Can you work these out from the model? Positions are in its coordinate system, mm. A direction names the side the tool comes from. Round coordinates to 2 decimals unless told otherwise and drop trailing zeros. Loops run counter-clockwise (first coordinate to the right, second up) from the corner with the lowest first, then second, coordinate; pieces in that order, holes last.
```python
from build123d import *

# Parameters (mm, degrees)
SKETCH4_W                      = 106
SKETCH4_H                      = 24
BOSS_EXTRUDE2_DEPTH            = 13
CUT_EXTRUDE3_START             = -9.7
SKETCH25_W                     = 106
SKETCH25_H                     = 8.1
CUT_EXTRUDE3_DEPTH             = 110.207903902
M5_CLEARANCE_HOLE1_D           = 5.5
SKETCH39_R                     = 4.2
CUT_EXTRUDE5_DEPTH             = 3.2
MIRROR3_START                  = -40.65
MIRROR3_OUTLINE_W              = 106
MIRROR3_OUTLINE_H              = 13
MIRROR3_OUTLINE_R              = 2.75
MIRROR3_DEPTH                  = 7.948683024
MIRROR3_START_2                = -24.601316976
MIRROR3_2_OUTLINE_W            = 106
MIRROR3_2_OUTLINE_H            = 13
MIRROR3_2_OUTLINE_R            = 4.2
MIRROR3_2_DEPTH                = 7.951316976
MIRROR3_START_3                = -32.701316976
MIRROR3_3_OUTLINE_W            = 106
MIRROR3_3_OUTLINE_H            = 3.3
MIRROR3_3_DEPTH                = 12.851316976
MIRROR3_4_OUTLINE_R            = 2.75
MIRROR3_4_DEPTH                = 4.751316976
M4_CLEARANCE_HOLE2_D           = 4.5
SKETCH31_W                     = 88
SKETCH31_H                     = 7
CUT_EXTRUDE4_DEPTH             = 7
SKETCH32_W                     = 6.6
SKETCH32_H                     = 7.948683024
BOSS_EXTRUDE3_DEPTH            = 10
SKETCH37_W                     = 6.6
SKETCH37_H                     = 7.948683024
BOSS_EXTRUDE4_DEPTH            = 10
M4_CLEARANCE_HOLE1_D           = 4.5
M4_CLEARANCE_HOLE1_ON_FACE_2_D = 4.5
SKETCH42_R                     = 4.75
CUT_EXTRUDE9_DEPTH             = 7
SKETCH43_R                     = 4.75
CUT_EXTRUDE10_DEPTH            = 7


# Read off the part's stored shape, not the designer's step: Mirror3
with BuildPart() as part:
    # Sketch4 → Boss-Extrude2 (new body)
    with BuildSketch(Plane.XY):
        with Locations((-36.891047602, -28.65)):
            Rectangle(SKETCH4_W, SKETCH4_H)
    extrude(amount=-BOSS_EXTRUDE2_DEPTH)

    # Sketch25 → Cut-Extrude3 (cut)
    with BuildSketch(Plane.XY.offset(CUT_EXTRUDE3_START)):
        with Locations((-36.891047602, -28.651316976)):
            Rectangle(SKETCH25_W, SKETCH25_H)
    extrude(amount=CUT_EXTRUDE3_DEPTH, mode=Mode.SUBTRACT)

    # M5 Clearance Hole1 (through all)
    with Locations(Plane(origin=(-74.391047602, -16.65, -5.55), x_dir=(0, 0, 1), z_dir=(0, 1, 0))):
        with Locations((0, 0), (0, 25), (0, 75), (0, 50)):
            Hole(M5_CLEARANCE_HOLE1_D / 2)

    # Sketch39 → Cut-Extrude5 (cut)
    with BuildSketch(Plane(origin=(0, -16.65, 0), x_dir=(1, 0, 0), z_dir=(0, 1, 0))):
        with Locations(Location((0.608952398, 5.55, 0), (0, 0, 270))):
            Circle(SKETCH39_R)
        with Locations(Location((-24.391047602, 5.55, 0), (0, 0, 270))):
            Circle(SKETCH39_R)
        with Locations(Location((-49.391047602, 5.55, 0), (0, 0, 270))):
            Circle(SKETCH39_R)
        with Locations(Location((-74.391047602, 5.55, 0), (0, 0, 270))):
            Circle(SKETCH39_R)
    extrude(amount=-CUT_EXTRUDE5_DEPTH, mode=Mode.SUBTRACT)

    # Mirror3 outline → Mirror3 (add)
    with BuildSketch(Plane(origin=(0, 0, 0), x_dir=(1, 0, 0), z_dir=(0, 1, 0)).offset(MIRROR3_START)):
        with Locations((-36.891047602, 19.5)):
            Rectangle(MIRROR3_OUTLINE_W, MIRROR3_OUTLINE_H)
        with Locations((0.608952398, 20.45)):
            Circle(MIRROR3_OUTLINE_R, mode=Mode.SUBTRACT)
        with Locations((-24.391047602, 20.45)):
            Circle(MIRROR3_OUTLINE_R, mode=Mode.SUBTRACT)
        with Locations((-49.391047602, 20.45)):
            Circle(MIRROR3_OUTLINE_R, mode=Mode.SUBTRACT)
        with Locations((-74.391047602, 20.45)):
            Circle(MIRROR3_OUTLINE_R, mode=Mode.SUBTRACT)
    extrude(amount=MIRROR3_DEPTH)

    # Mirror3 2 outline → Mirror3 2 (add)
    with BuildSketch(Plane(origin=(0, 0, 0), x_dir=(1, 0, 0), z_dir=(0, 1, 0)).offset(MIRROR3_START_2)):
        with Locations((-36.891047602, 19.5)):
            Rectangle(MIRROR3_2_OUTLINE_W, MIRROR3_2_OUTLINE_H)
        with Locations((0.608952398, 20.45)):
            Circle(MIRROR3_2_OUTLINE_R, mode=Mode.SUBTRACT)
        with Locations((-24.391047602, 20.45)):
            Circle(MIRROR3_2_OUTLINE_R, mode=Mode.SUBTRACT)
        with Locations((-49.391047602, 20.45)):
            Circle(MIRROR3_2_OUTLINE_R, mode=Mode.SUBTRACT)
        with Locations((-74.391047602, 20.45)):
            Circle(MIRROR3_2_OUTLINE_R, mode=Mode.SUBTRACT)
    extrude(amount=MIRROR3_2_DEPTH)

    # Mirror3 3 outline → Mirror3 3 (add)
    with BuildSketch(Plane(origin=(0, 0, 0), x_dir=(1, 0, 0), z_dir=(0, 1, 0)).offset(MIRROR3_START_3)):
        with Locations((-36.891047602, 14.65)):
            Rectangle(MIRROR3_3_OUTLINE_W, MIRROR3_3_OUTLINE_H)
    extrude(amount=MIRROR3_3_DEPTH)

    # Mirror3 4 outline → Mirror3 4 (add)
    # profile 1 of 4: a face of its own
    with BuildSketch(Plane(origin=(0, 0, 0), x_dir=(1, 0, 0), z_dir=(0, 1, 0)).offset(MIRROR3_START_2)):
        with BuildLine():
            Line((-0.037190001, 16.3), (1.255094797, 16.3))
            ThreePointArc((1.255094797, 16.3), (0.608952398, 24.65), (-0.037190001, 16.3))
        make_face()
        with Locations((0.608952398, 20.45)):
            Circle(MIRROR3_4_OUTLINE_R, mode=Mode.SUBTRACT)
    # profile 2 of 4: a face of its own
    with BuildSketch(Plane(origin=(0, 0, 0), x_dir=(1, 0, 0), z_dir=(0, 1, 0)).offset(MIRROR3_START_2)):
        with BuildLine():
            ThreePointArc((-73.744905203, 16.3), (-74.391047602, 24.65), (-75.037190001, 16.3))
            Line((-75.037190001, 16.3), (-73.744905203, 16.3))
        make_face()
        with Locations((-74.391047602, 20.45)):
            Circle(MIRROR3_4_OUTLINE_R, mode=Mode.SUBTRACT)
    # profile 3 of 4: a face of its own
    with BuildSketch(Plane(origin=(0, 0, 0), x_dir=(1, 0, 0), z_dir=(0, 1, 0)).offset(MIRROR3_START_2)):
        with BuildLine():
            Line((-25.037190001, 16.3), (-23.744905203, 16.3))
            ThreePointArc((-23.744905203, 16.3), (-24.391047602, 24.65), (-25.037190001, 16.3))
        make_face()
        with Locations((-24.391047602, 20.45)):
            Circle(MIRROR3_4_OUTLINE_R, mode=Mode.SUBTRACT)
    # profile 4 of 4: a face of its own
    with BuildSketch(Plane(origin=(0, 0, 0), x_dir=(1, 0, 0), z_dir=(0, 1, 0)).offset(MIRROR3_START_2)):
        with BuildLine():
            ThreePointArc((-48.744905203, 16.3), (-49.391047602, 24.65), (-50.037190001, 16.3))
            Line((-50.037190001, 16.3), (-48.744905203, 16.3))
        make_face()
        with Locations((-49.391047602, 20.45)):
            Circle(MIRROR3_4_OUTLINE_R, mode=Mode.SUBTRACT)
    extrude(amount=MIRROR3_4_DEPTH)

    # M4 Clearance Hole2 (through all)
    with Locations(Plane(origin=(11.108952398, -40.65, -13), x_dir=(0, 0, -1), z_dir=(0, -1, 0))):
        with Locations((0, 0), (0, -96)):
            Hole(M4_CLEARANCE_HOLE2_D / 2)

    # Sketch31 → Cut-Extrude4 (cut)
    with BuildSketch(Plane(origin=(0, -16.65, 0), x_dir=(1, 0, 0), z_dir=(0, 1, 0))):
        with Locations((-36.891047602, 13)):
            Rectangle(SKETCH31_W, SKETCH31_H)
    extrude(amount=-CUT_EXTRUDE4_DEPTH, mode=Mode.SUBTRACT)

    # Sketch32 → Boss-Extrude3 (add)
    with BuildSketch(Plane.ZY.offset(89.891047602)):
        with Locations((-13, -36.675658488)):
            Rectangle(SKETCH32_W, SKETCH32_H)
    extrude(amount=BOSS_EXTRUDE3_DEPTH)

    # Sketch37 → Boss-Extrude4 (add)
    with BuildSketch(Plane(origin=(16.108952398, 0, 0), x_dir=(0, 0, -1), z_dir=(1, 0, 0))):
        with Locations((13, -36.675658488)):
            Rectangle(SKETCH37_W, SKETCH37_H)
    extrude(amount=BOSS_EXTRUDE4_DEPTH)

    # M4 Clearance Hole1 (through all)
    with Locations(Plane(origin=(-95.541407791, -40.65, -13), x_dir=(0, 0, -1), z_dir=(0, -1, 0))):
        with Locations((0, 0), (0, 117.300360189)):
            Hole(M4_CLEARANCE_HOLE1_D / 2)

    # M4 Clearance Hole1 on face 2 (through all)
    with Locations(Plane(origin=(38.237961727, 0, -11.003941324), x_dir=(0, 0, -1), z_dir=(0, -1, 0))):
        with Locations((0, 0)):
            Hole(M4_CLEARANCE_HOLE1_ON_FACE_2_D / 2)

    # Sketch42 → Cut-Extrude9 (cut)
    with BuildSketch(Plane(origin=(0, -16.65, 0), x_dir=(1, 0, 0), z_dir=(0, 1, 0))):
        with Locations((11.108952398, 13)):
            Circle(SKETCH42_R)
    extrude(amount=-CUT_EXTRUDE9_DEPTH, mode=Mode.SUBTRACT)

    # Sketch43 → Cut-Extrude10 (cut)
    with BuildSketch(Plane(origin=(0, -16.65, 0), x_dir=(1, 0, 0), z_dir=(0, 1, 0))):
        with Locations((-84.891047602, 13)):
            Circle(SKETCH43_R)
    extrude(amount=-CUT_EXTRUDE10_DEPTH, mode=Mode.SUBTRACT)


solid = part.part
```
(1) If I drill on line 1 (X direction, y = -21.3, z = -20.45); line 2 (Y direction, x = -3.5, z = -24), over which ranges is the centre line in solid material (lowest first)?
(2) Suppose I cut it at B-B (x = -17). Write out the boundary of the cut face in (y, z), then the cut area to 3 significant figures.
(3) We'd pull the mould along X, two halves only. Please class faces 4 (the flat face through (-38, -32.701, -5)), 5 (the flat face through (16.109, -23, -13)), 6 (the cylindrical face through (0.445, -18.228, -1.353)): released by +X, released by -X, zero draft, split by the parting line, or undercut.
(4) For pin 1 (7 mm diameter, centred on x = 0.61, z = -20.45, fed in from +Y); pin 2 (1 mm diameter, centred on y = -19.5, z = -5, fed in from +X); pin 3 (7 mm diameter, centred on x = -95.54, z = -13, fed in from +Y), each with a flat end and sliding along its axis, tell me the tip position at first contact or that it passes through.
(5) Which directions (+Z, -Z, +X, -X, +Y, -Y) give clear straight access to the entire face, cutting with the end or side of a thin tool? Please do faces 1 (the flat face through (-38, -40.65, -13)), 2 (the flat face through (-38, -20, -16.5)), 3 (the flat face through (-38, -29, -16.3)).
(6) Suppose I cut it at C-C (y = -26.25). Write out the boundary of the cut face in (x, z), then the cut area to 3 significant figures.
(7) Suppose I cut it at D-D (z = -20.45). Give the number of separate pieces and of enclosed holes in the cut face, then the cut area to 3 significant figures.
(8) Suppose I cut it at A-A (z = -13). Write out the boundary of the cut face in (x, y).
Check result:
1. line 1: x = -89.89 to -77.14, -71.64 to -52.14, -46.64 to -27.14, -21.64 to -2.14, 3.36 to 16.11
1. line 2: y = -40.65 to -32.7, -24.6 to -16.65
2. outline: (-40.65, -26) - (-32.7, -26) - (-32.7, -16.3) - (-24.6, -16.3) - (-24.6, -26) - (-16.65, -26) - (-16.65, -16.5) - (-23.65, -16.5) - (-23.65, -9.5) - (-16.65, -9.5) - (-16.65, 0) - (-24.6, 0) - (-24.6, -9.7) - (-32.7, -9.7) - (-32.7, 0) - (-40.65, 0) - close
2. area: 418 mm2
3. face 4: zero draft
3. face 5: released by +X
3. face 6: undercut
4. pin 1: stops at y = -19.85
4. pin 2: stops at x = 16.11
4. pin 3: stops at y = -32.7
5. face 1: +Z, -Z, +X, -X, -Y
5. face 2: +Y
5. face 3: -Z, +X, -X
6. outline: (-89.89, -16.3) - (16.11, -16.3) - (16.11, -9.7) - (-89.89, -9.7) - close; hole circle Ø4.5 at (-84.89, -13); hole circle Ø4.5 at (11.11, -13)
6. area: 668 mm2
7. separate pieces: 10
7. enclosed holes: 0
7. area: 1,300 mm2
8. outline: (-99.89, -40.65) - (-97.79, -40.65) - (-97.79, -32.7) - (-99.89, -32.7) - close; (-93.29, -40.65) - (-87.14, -40.65) - (-87.14, -23.65) - (-89.64, -23.65) - (-89.64, -16.65) - (-89.89, -16.65) - (-89.89, -32.7) - (-93.29, -32.7) - close; (-82.64, -40.65) - (8.86, -40.65) - (8.86, -23.65) - (-82.64, -23.65) - close; (13.36, -40.65) - (19.51, -40.65) - (19.51, -32.7) - (16.11, -32.7) - (16.11, -16.65) - (15.86, -16.65) - (15.86, -23.65) - (13.36, -23.65) - close; (24.01, -40.65) - (26.11, -40.65) - (26.11, -32.7) - (24.01, -32.7) - close
